Autodesk Inventor part; units mm, degrees
ref_plane "YZ Plane" through (0, 0, 0) normal (1, 0, 0) x (0, 1, 0)
ref_plane "XZ Plane" through (0, 0, 0) normal (0, 1, 0) x (-1, 0, 0)
ref_plane "XY Plane" through (0, 0, 0) normal (0, 0, 1) x (1, 0, 0)
sketch "Sketch1" plane through (0, 0, 0) normal (0, 0, 1) x (1, 0, 0)
  line L0 (0, 0) -> (195.58, 0)
  line L1 (195.58, 0) -> (195.58, 9.525)
  line L2 (195.58, 9.525) -> (0, 9.525)
  line L3 (0, 9.525) -> (0, 0)
  dimension "d0" = 9.525
  dimension "d1" = 195.58
extrude "Extrusion1" add sketch "Sketch1" along normal blind 9.525
sketch "Sketch2" plane through (0, 9.525, 0) normal (0, 1, 0) x (1, 0, 0)
  line L0 (195.58, 0) -> (0, 0)
  line L1 (9.525, 0) -> (9.525, -9.525)
  line L2 (73.66, -9.525) -> (73.66, 0)
  line L3 (83.185, 0) -> (83.185, -9.525)
  line L4 (112.395, 0) -> (112.395, -9.525)
  line L5 (121.92, -9.525) -> (121.92, 0)
  line L6 (186.055, 0) -> (186.055, -9.525)
  point P0 (4.7625, -4.7625)
  point P1 (78.4225, -4.7625)
  point P2 (117.1575, -4.7625)
  point P3 (190.8175, -4.7625)
  dimension "d4" = 4.7625
  dimension "d5" = 4.7625
  dimension "d6" = 4.7625
  dimension "d7" = 4.7625
  dimension "d8" = 4.7625
  dimension "d9" = 4.7625
  dimension "d10" = 4.7625
  dimension "d11" = 4.7625
hole "Hole1" at (4.7625, 9.525, 4.7625) at (78.4225, 9.525, 4.7625) at (117.1575, 9.525, 4.7625) at (190.8175, 9.525, 4.7625) direction (0, -1, 0) diameter 4.4958 end through all countersink diameter 8.4328 countersink angle 82
properties part number "SupportBar" material "Aluminum-6061"
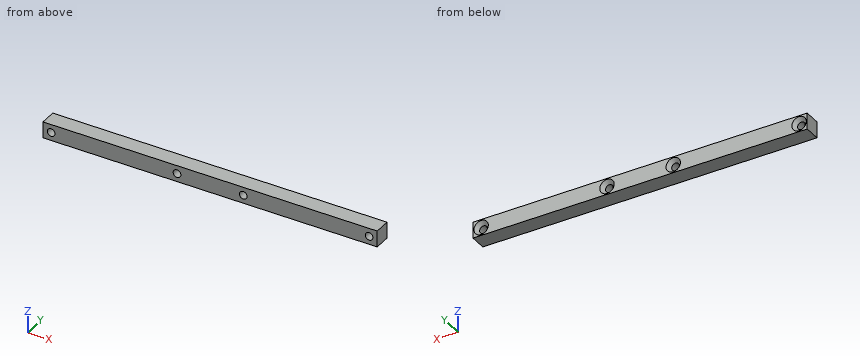
Verification items for the finished model (mm, model axes). Give positions to 0.01 mm unless a question says otherwise; leave off trailing zeros. Write each loop counter-clockwise with the first axis right and the second up, starting at its lowest first coordinate (ties: lowest second). Pieces come first, ordered by that corner, then holes. Notation, with made-up numbers: (-36, -31) - (7, -31) arc R17 ccw to (7, -22) - close; hole circle Ø10 at (82, 37.5). An arc over 180 degrees is marked (long way). Put each result on its own line as item: value.
Q1. Section check A-A on y = 2.75. Record the cut outline in (x, z) (1 decimal).
Result:
outline: (0, 0) - (195.6, 0) - (195.6, 9.5) - (0, 9.5) - close; hole circle Ø4.5 at (4.8, 4.8); hole circle Ø4.5 at (78.4, 4.8); hole circle Ø4.5 at (117.2, 4.8); hole circle Ø4.5 at (190.8, 4.8)
Q2. Depth check by flat-ended pin: P1, Ø1.5, axis at y = 5.5, z = 2.5, coming from the -X side; P2, Ø3.5, axis at x = 117.16, z = 4.76, coming from the -Y side; P3, Ø3, axis at x = 80.5, z = 5, coming from the +Y side. Enter the tip coordinate at first touch or a pass-through.
Result:
P1: x = 0
P2: through
P3: y = 8.81
Q3. Section check B-B on z = 4. Count the separate pieces of the cut face and the enclosed holes in it, and give its area (3 significant figures).
Result:
separate pieces: 5
enclosed holes: 0
area: 1,680 mm2
Q4. Scan lines: probe 1 along X at (y, z) = (8.75, 3.5); probe 2 along X at (y, z) = (0.5, 5.5); probe 3 along Z at (x, y) = (76.5, 6.5) (3 decimals). Record each from-to range of solid material in increasing order. Write a range as from..to.
Result:
probe 1: 0..1.45, 8.07..75.11, 81.73..113.85, 120.47..187.51, 194.13..195.58
probe 2: 0..2.64, 6.89..76.3, 80.55..115.03, 119.28..188.69, 192.94..195.58
probe 3: 0..3.598, 5.927..9.525
